from build123d import *

# Parameters (mm, degrees)
CHANFREIN1_SIZE    = 0.2
CHANFREIN2_SIZE    = 0.5
CHANFREIN3_SIZE    = 0.2
ESQUISSE2_R        = 10
BOSS_EXTRU_1_DEPTH = 0.5
CONG_1_R           = 1
CONG_2_R           = 0.2
ECHELLE1_SCALE     = 10


with BuildPart() as part:
    # Esquisse1 → Révolution1 (revolve)
    with BuildSketch(Plane.XY, mode=Mode.PRIVATE) as r_volution1_sk:
        with BuildLine():
            Line((0, 0), (0, 50))
            Line((0, 50), (0, 52))
            Line((0, 52), (-2, 52))
            ThreePointArc((-2, 52), (-2.299732451, 51.712667184), (-2.025311774, 51.401069717))
            Line((-2.025311774, 51.401069717), (-2.025311774, 49.792758152))
            ThreePointArc((-2.025311774, 49.792758152), (-7.754131729, 46.314542037), (-10, 40))
            Line((-10, 40), (-10, 0))
            Line((-10, 0), (-8.354852758, 0))
            Line((-8.354852758, 0), (-8.354852758, 0.3))
            Line((-8.354852758, 0.3), (-7.354852758, 0.3))
            Line((-7.354852758, 0.3), (-7.354852758, 0))
            Line((-7.354852758, 0), (-6.354852758, 0))
            Line((-6.354852758, 0), (-6.354852758, 0.3))
            Line((-6.354852758, 0.3), (-5.354852758, 0.3))
            Line((-5.354852758, 0.3), (-5.354852758, 0))
            Line((-5.354852758, 0), (-2.025311774, 0))
            Line((-2.025311774, 0), (-2.025311774, 0.3))
            Line((-2.025311774, 0.3), (-1.025311774, 0.3))
            Line((-1.025311774, 0.3), (-1.025311774, 0))
            Line((-1.025311774, 0), (0, 0))
        make_face()
    revolve(r_volution1_sk.sketch.rotate(Axis((0, 0, 0), (0, 1, 0)), 180), axis=Axis((0, 0, 0), (0, 1, 0)))

    # Chanfrein1
    chanfrein1_edges = [part.edges().sort_by_distance(p)[0] for p in [
        (-1.025311774, 0, 0),
        (-2.025311774, 0, 0),
        (-5.354852758, 0, 0),
        (-6.354852758, 0, 0),
        (-7.354852758, 0, 0),
        (-8.354852758, 0, 0),
    ]]
    chamfer(chanfrein1_edges, length=CHANFREIN1_SIZE)

    # Chanfrein2
    chanfrein2_edges = [part.edges().sort_by_distance(p)[0] for p in [
        (-10, 0, 0),
    ]]
    chamfer(chanfrein2_edges, length=CHANFREIN2_SIZE)

    # Coque2: read off the stored shape, not the designer's step
    # Coque2 outline → Coque2 (revolve, cut)
    with BuildSketch(Plane.XY):
        with BuildLine():
            Line((8.854852758, 0.8), (8.854852758, 0.5))
            Line((8.854852758, 0.5), (9.292893219, 0.5))
            Line((9.292893219, 0.5), (9.5, 0.707106781))
            Line((9.5, 0.707106781), (9.5, 39.999999997))
            ThreePointArc((9.5, 39.999999997), (7.236727916, 46.154654261), (1.525311771, 49.376749117))
            Line((1.525311771, 49.376749117), (1.525311774, 52))
            Line((1.525311774, 52), (0, 52))
            Line((0, 52), (0, 0.5))
            Line((0, 0.5), (0.525311774, 0.5))
            Line((0.525311774, 0.5), (0.525311774, 0.8))
            Line((0.525311774, 0.8), (2.525311774, 0.8))
            Line((2.525311774, 0.8), (2.525311774, 0.5))
            Line((2.525311774, 0.5), (4.854852758, 0.5))
            Line((4.854852758, 0.5), (4.854852758, 0.8))
            Line((4.854852758, 0.8), (8.854852758, 0.8))
        make_face()
    revolve(axis=Axis((0, 0, 0), (0, 1, 0)), mode=Mode.SUBTRACT)

    # Chanfrein3
    # the kernel refuses this chamfer: 0.25748488, 0.2 mm, written as the material it adds along each edge
    with BuildSketch(Plane(origin=(0, 49.792758152, 0), x_dir=(1, 0, 0), z_dir=(0, 0, 1))) as chanfrein3_piece_1:
        with BuildLine():
            Line((2.281904858, -0.056593084), (2.025311774, CHANFREIN3_SIZE))
            Line((2.025311774, CHANFREIN3_SIZE), (2.025311774, 0))
            ThreePointArc((2.025311774, 0), (2.158033883, -0.028389777), (2.281904858, -0.056593084))
        make_face()
    revolve(axis=Axis((0, 49.792758152, 0), (0, 1, 0)))

    # Esquisse2 → Boss.-Extru.1 (add)
    with BuildSketch(Plane(origin=(0, 0.5, 0), x_dir=(1, 0, 0), z_dir=(0, 1, 0))):
        Circle(ESQUISSE2_R)
    extrude(amount=BOSS_EXTRU_1_DEPTH)

    # Congé1
    cong_1_edges = [part.edges().sort_by_distance(p)[0] for p in [
        (-9.5, 1, 0),
    ]]
    fillet(cong_1_edges, radius=CONG_1_R)

    # Congé2
    cong_2_edges = [part.edges().sort_by_distance(p)[0] for p in [
        (-1.525311771, 49.376749117, 0),
    ]]
    fillet(cong_2_edges, radius=CONG_2_R)


with BuildPart() as part_1:
    # Echelle1: scaled about (0, 0, 0)
    add(part.part.scale(ECHELLE1_SCALE))


solid = part_1.part
Can you work these out from the model? Positions are in its coordinate system, mm. A direction names the side the tool comes from. Give positions to 0.01 mm unless a question says otherwise; leave off trailing zeros. Order: outer loops, then holes, each group sorted by start corner. A loop starts at its lowest first (then second) coordinate and runs counter-clockwise, first axis right, second up. Notation, with made-up numbers: M 45.5,41.5 L 53.5,41.5 A11 ccw 53.5,59.5 Z; hole C 67.5,64.5 d8. An arc over 180 degrees is marked long. Use a Markdown table: item, result. Add a question column.
Item 1: Will these pins go through, and if not, where does the flat tip stop? pin 1 (6 mm diameter, centred on y = 460, z = -3.5, fed in from -X); pin 2 (12 mm diameter, centred on y = 344, z = -16, fed in from +X); pin 3 (8 mm diameter, centred on x = 22.5, z = -78.5, fed in from +Y).
Item 2: We'd pull the mould along X, two halves only. Please class faces 1 (the cylindrical face through (95.38, 199.74, -30.04)), 2 (the flat face through (5, 520, 15)), 3 (the cylindrical face through (51.076, 2.493, -16.085)): +X half, -X half, draft (parallel to the pull), parting line (faces both ways), or undercut.
Item 3: If I drill on L1, parallel to X at y = 505, z = 0; L2, parallel to X at y = 439.5, z = 46; L3, parallel to Z at x = -24, y = 160.5, over which ranges is the centre line in solid material (lowest first)? Write a range as [from, to].
Item 4: Suppose I cut it at A-A (y = 35). List the corners of the cut face in (x, z) for me, then the cut area to 3 significant figures.
Item 5: For faces 4 (the cylindrical face through (-2.22, 2.49, 10.01)), 5 (the flat face through (-78, 0, -36)), 6 (the cylindrical face through (-3.31, 507.9, 14.89)), 7 (the flat face through (-1, 10, -1)), which set-ups out of +Z, -Z, +X, -X, +Y, -Y let a thin tool reach every point of the face, with its end or its side?
Answer sheet:
| question | item | result |
|---|---|---|
| 1 | pin 1 | stops at x = -82.09 |
| 1 | pin 2 | stops at x = 99.5 |
| 1 | pin 3 | stops at y = 463 |
| 2 | face 1 | parting line |
| 2 | face 2 | draft |
| 2 | face 3 | undercut |
| 3 | L1 | x = [-20.25, -15.25], [15.25, 20.25] |
| 3 | L2 | x = [-79.52, -73.14], [73.14, 79.52] |
| 3 | L3 | z = [-97.08, -91.92], [91.92, 97.08] |
| 4 | outline | C 0,0 d200; hole C 0,0 d190 |
| 4 | area | 3,060 mm² |
| 5 | face 4 | -Y |
| 5 | face 5 | +Z, -Z, +X, -X, -Y |
| 5 | face 6 | +Y |
| 5 | face 7 | none |
